```python
from build123d import *

# Parameters (mm, degrees)
BOSS_EXTRUDE3_DEPTH = 10
SKETCH3_R           = 4
CUT_EXTRUDE3_DEPTH  = 14.0462
CUT_EXTRUDE4_DEPTH  = 3
MIRROR1_START       = 7
MIRROR1_DEPTH       = 3
MIRROR1_2_DEPTH     = 7
MIRROR1_3_DEPTH     = 3


# Read off the part's stored shape, not the designer's step: Mirror1
with BuildPart() as part:
    # Sketch1 → Boss-Extrude3 (new body)
    with BuildSketch(Plane.YZ):
        with BuildLine():
            Line((-28.968617751, -12.789334175), (28.968617751, -12.789334175))
            ThreePointArc((28.968617751, -12.789334175), (44.579120821, 0), (35.110840206, 17.821518929))
            ThreePointArc((35.110840206, 17.821518929), (30.644623053, 21.505675602), (28.968617751, 27.047436358))
            Line((28.968617751, 27.047436358), (28.968617751, 39.053986921))
            ThreePointArc((28.968617751, 39.053986921), (26.039685563, 46.125054733), (18.968617751, 49.053986921))
            Line((18.968617751, 49.053986921), (-18.968617751, 49.053986921))
            ThreePointArc((-18.968617751, 49.053986921), (-26.039685563, 46.125054733), (-28.968617751, 39.053986921))
            Line((-28.968617751, 39.053986921), (-28.968617751, 27.047436358))
            ThreePointArc((-28.968617751, 27.047436358), (-30.644623053, 21.505675602), (-35.110840206, 17.821518929))
            ThreePointArc((-35.110840206, 17.821518929), (-44.579120821, 0), (-28.968617751, -12.789334175))
        make_face()
    extrude(amount=BOSS_EXTRUDE3_DEPTH)

    # Sketch3 → Cut-Extrude3 (cut)
    with BuildSketch(Plane.YZ.offset(10)):
        with Locations(Location((0, 3.132326373, 0), (0, 0, 270))):
            Circle(SKETCH3_R)
    extrude(amount=-CUT_EXTRUDE3_DEPTH, mode=Mode.SUBTRACT)

    # Sketch4 → Cut-Extrude4 (cut)
    with BuildSketch(Plane.YZ.offset(10)):
        with BuildLine():
            Line((-12.95, 49.053986921), (-12.95, 31.267703884))
            ThreePointArc((-12.95, 31.267703884), (0, 18.317703884), (12.95, 31.267703884))
            Line((12.95, 31.267703884), (12.95, 49.053986921))
            Line((12.95, 49.053986921), (-12.95, 49.053986921))
        make_face()
    extrude(amount=-CUT_EXTRUDE4_DEPTH, mode=Mode.SUBTRACT)

    # Mirror1 outline → Mirror1 (cut)
    with BuildSketch(Plane.YZ.offset(MIRROR1_START)):
        with BuildLine():
            ThreePointArc((4.30437196, -12.789334175), (0, -12.053051137), (-4.30437196, -12.789334175))
            Line((-4.30437196, -12.789334175), (4.30437196, -12.789334175))
        make_face()
    extrude(amount=MIRROR1_DEPTH, mode=Mode.SUBTRACT)

    # Mirror1 2 outline → Mirror1 2 (add)
    with BuildSketch(Plane.YZ):
        with BuildLine():
            ThreePointArc((-28.968617751, -32.789334175), (-26.039685563, -39.860401987), (-18.968617751, -42.789334175))
            Line((-18.968617751, -42.789334175), (18.968617751, -42.789334175))
            ThreePointArc((18.968617751, -42.789334175), (26.039685563, -39.860401987), (28.968617751, -32.789334175))
            Line((28.968617751, -32.789334175), (28.968617751, -20.782783611))
            ThreePointArc((28.968617751, -20.782783611), (30.644623053, -15.241022855), (35.110840206, -11.556866182))
            ThreePointArc((35.110840206, -11.556866182), (32.100944124, -12.478176697), (28.968617751, -12.789334175))
            Line((28.968617751, -12.789334175), (-28.968617751, -12.789334175))
            ThreePointArc((-28.968617751, -12.789334175), (-32.100944124, -12.478176697), (-35.110840206, -11.556866182))
            ThreePointArc((-35.110840206, -11.556866182), (-30.644623053, -15.241022855), (-28.968617751, -20.782783611))
            Line((-28.968617751, -20.782783611), (-28.968617751, -32.789334175))
        make_face()
    extrude(amount=MIRROR1_2_DEPTH)

    # Mirror1 3 outline → Mirror1 3 (add)
    with BuildSketch(Plane.YZ.offset(MIRROR1_START)):
        with BuildLine():
            ThreePointArc((-28.968617751, -32.789334175), (-26.039685563, -39.860401987), (-18.968617751, -42.789334175))
            Line((-18.968617751, -42.789334175), (-12.95, -42.789334175))
            Line((-12.95, -42.789334175), (-12.95, -25.003051137))
            ThreePointArc((-12.95, -25.003051137), (-10.569865583, -17.521043281), (-4.30437196, -12.789334175))
            Line((-4.30437196, -12.789334175), (-28.968617751, -12.789334175))
            ThreePointArc((-28.968617751, -12.789334175), (-32.100944124, -12.478176697), (-35.110840206, -11.556866182))
            ThreePointArc((-35.110840206, -11.556866182), (-30.644623053, -15.241022855), (-28.968617751, -20.782783611))
            Line((-28.968617751, -20.782783611), (-28.968617751, -32.789334175))
        make_face()
        with BuildLine():
            Line((12.95, -25.003051137), (12.95, -42.789334175))
            Line((12.95, -42.789334175), (18.968617751, -42.789334175))
            ThreePointArc((18.968617751, -42.789334175), (26.039685563, -39.860401987), (28.968617751, -32.789334175))
            Line((28.968617751, -32.789334175), (28.968617751, -20.782783611))
            ThreePointArc((28.968617751, -20.782783611), (30.644623053, -15.241022855), (35.110840206, -11.556866182))
            ThreePointArc((35.110840206, -11.556866182), (32.100944124, -12.478176697), (28.968617751, -12.789334175))
            Line((28.968617751, -12.789334175), (4.30437196, -12.789334175))
            ThreePointArc((4.30437196, -12.789334175), (10.569865583, -17.521043281), (12.95, -25.003051137))
        make_face()
        with BuildLine():
            ThreePointArc((-4.304371959, 19.053986921), (0, 18.317703884), (4.304371959, 19.053986921))
            Line((4.304371959, 19.053986921), (-4.304371959, 19.053986921))
        make_face()
    extrude(amount=MIRROR1_3_DEPTH)


solid = part.part
```
For this review, take the finished solid that the model builds, in its own axes (mm). A direction names the side the tool comes from. Round coordinates to 2 decimals unless told otherwise and drop trailing zeros. Write each loop counter-clockwise with the first axis right and the second up, starting at its lowest first coordinate (ties: lowest second). Pieces come first, ordered by that corner, then holes. Notation, with made-up numbers: (-27, 28) - (-21, 28) arc R9 cw to (-21, 43) - close; hole circle Ø6 at (-27, -31). An arc over 180 degrees is marked (long way). Answer as a JSON object with one key per item and string values.
1. We need section B-B on x = 4.5. Give the boundary of the cut face in (y, z), then the cut area to 3 significant figures.
Response values:
{"outline": "(-35.11, -11.56) arc R10 cw to (-28.97, -20.78) - (-28.97, -32.79) arc R10 ccw to (-18.97, -42.79) - (18.97, -42.79) arc R10 ccw to (28.97, -32.79) - (28.97, -20.78) arc R10 cw to (35.11, -11.56) arc R15.92 ccw to (35.11, 17.82) arc R10 cw to (28.97, 27.05) - (28.97, 39.05) arc R10 ccw to (18.97, 49.05) - (-18.97, 49.05) arc R10 ccw to (-28.97, 39.05) - (-28.97, 27.05) arc R10 cw to (-35.11, 17.82) arc R15.92 ccw to start; hole circle Ø8 at (0, 3.13)", "area": "6,020 mm2"}
2. For pin 1 Ø0.9 at (x, y) = (9, 0.5) entering from +Z; pin 2 Ø3.5 at (x, z) = (8, -29.5) entering from +Y; pin 3 Ø2 at (x, y) = (3.5, -21) entering from +Z, all flat-tipped, find the tip position at first contact; note any pin that passes through.
Response values:
{"pin 1": "stops at z = 19.05", "pin 2": "stops at y = 28.97", "pin 3": "stops at z = 49"}
3. Tool access review of faces 1 (the face through (5, -28.969, 33)), 2 (the face through (5, 28.969, -27)), 3 (the face through (8, -12.95, -34)), 4 (the face through (8.521, -10.634, 23.877)): name each direction out of +Z, -Z, +X, -X, +Y, -Y from which nothing blocks a thin tool from reaching the whole face with its end or side.
Response values:
{"face 1": "+Z, +X, -X, -Y", "face 2": "-Z, +X, -X, +Y", "face 3": "-Z, +X", "face 4": "+Z, +X"}
4. We need section D-D on y = 11.5. Give the boundary of the cut face in (x, z).
Response values:
{"outline": "(0, -42.79) - (7, -42.79) - (7, -19.05) - (10, -19.05) - (10, 25.31) - (7, 25.31) - (7, 49.05) - (0, 49.05) - close"}
5. To check wall thickness, follow line 1 along X through (y, z) = (1, 45); line 2 along Y through (x, z) = (8.25, 35.5); line 3 along Y through (x, z) = (1, -30). State the ranges of each line that lie inside material, in increasing order.
Response values:
{"line 1": "x = 0 to 7", "line 2": "y = -28.97 to -12.95, 12.95 to 28.97", "line 3": "y = -28.97 to 28.97"}
6. Draft analysis for pull direction Y (two halves, no side actions). For faces 5 (the face through (4, 0, -42.789)), 6 (the face through (9, 12.95, 40)), 7 (the face through (4.9, 26, -39.9)), state which applies: +Y half, -Y half, draft (parallel to the pull), parting line (faces both ways), or undercut.
Response values:
{"face 5": "draft", "face 6": "undercut", "face 7": "+Y half"}
7. We need section C-C on z = -31. Give the boundary of the cut face in (x, y), then the cut area to 3 significant figures.
Response values:
{"outline": "(0, -28.97) - (10, -28.97) - (10, -12.95) - (7, -12.95) - (7, 12.95) - (10, 12.95) - (10, 28.97) - (0, 28.97) - close", "area": "502 mm2"}
8. We need section A-A on y = 0. Give the boundary of the cut face in (x, z), then the cut area to 3 significant figures.
Response values:
{"outline": "(0, -42.79) - (7, -42.79) - (7, -12.05) - (10, -12.05) - (10, -0.87) - (0, -0.87) - close; (0, 7.13) - (10, 7.13) - (10, 19.05) - (7, 19.05) - (7, 49.05) - (0, 49.05) - close", "area": "656 mm2"}
